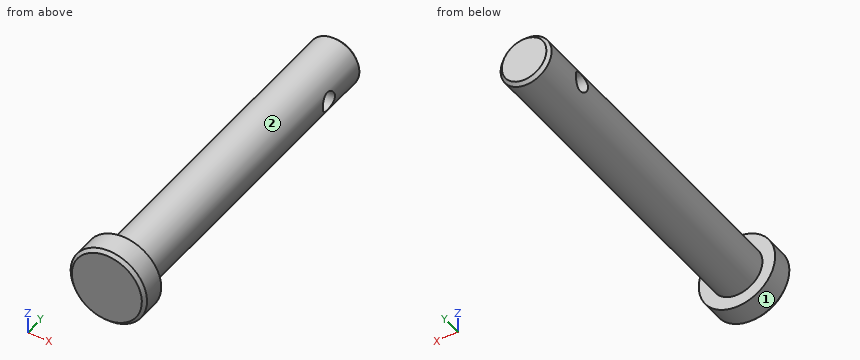
```python
from build123d import *

# Parameters (mm, degrees)
SKETCH1_R               = 12
BOSS_EXTRUDE1_DEPTH     = 8
CHAMFER1_SIZE           = 1
SKETCH2_R               = 8
BOSS_EXTRUDE2_DEPTH     = 105
CHAMFER2_SIZE           = 1
CUT_EXTRUDE1_DEPTH      = 115.267230648
CUT_EXTRUDE1_DEPTH_BACK = 115.267230648
SKETCH3_R               = 3


with BuildPart() as part:
    # Sketch1 → Boss-Extrude1 (new body)
    with BuildSketch(Plane(origin=(0, 0, 0), x_dir=(-1, 0, 0), z_dir=(0, 1, 0))):
        with Locations(Location((0, 0, 0), (0, 0, 90))):
            Circle(SKETCH1_R)
    extrude(amount=BOSS_EXTRUDE1_DEPTH)

    # Chamfer1
    chamfer1_edges = [part.edges().sort_by_distance(p)[0] for p in [
        (0, 0, -12),
    ]]
    chamfer(chamfer1_edges, length=CHAMFER1_SIZE)

    # Sketch2 → Boss-Extrude2 (add)
    with BuildSketch(Plane(origin=(0, 8, 0), x_dir=(-1, 0, 0), z_dir=(0, 1, 0))):
        with Locations(Location((0, 0, 0), (0, 0, 90))):
            Circle(SKETCH2_R)
    extrude(amount=BOSS_EXTRUDE2_DEPTH)

    # Chamfer2
    chamfer2_edges = [part.edges().sort_by_distance(p)[0] for p in [
        (0, 113, -8),
    ]]
    chamfer(chamfer2_edges, length=CHAMFER2_SIZE)

    # Sketch3 → Cut-Extrude1 (cut, two sides: drawn at the far end of the back side and taken through both)
    with BuildSketch(Plane.YZ.offset(-CUT_EXTRUDE1_DEPTH_BACK)):
        with Locations(Location((97, 0, 0), (0, 0, 270))):
            Circle(SKETCH3_R)
    extrude(amount=CUT_EXTRUDE1_DEPTH + CUT_EXTRUDE1_DEPTH_BACK, mode=Mode.SUBTRACT)


solid = part.part
```
Work out the finished part from the listing and answer in its coordinate system (mm). Face numbers are marked on the shaded views. A direction names the side the tool comes from. Give positions to 0.01 mm unless a question says otherwise; leave off trailing zeros. Loops run counter-clockwise (first coordinate to the right, second up) from the corner with the lowest first, then second, coordinate; pieces in that order, holes last. Notation, with made-up numbers: (7.25, 30) -> (16.25, 30) arc R31 cw to (16.25, 58) -> close; hole circle Ø3 at (-34, 42.25). An arc over 180 degrees is marked (long way). Use CSV: the item, a comma, the result in double quotes.
1. The part is cut by section C-C (y = 97). Write down the section's boundary in (x, z).
Found:
outline,"(-7.42, -3) arc R8 ccw to (7.42, -3) -> close; (-7.42, 3) -> (7.42, 3) arc R8 ccw to start"
2. Flat-ended cylindrical pins translate along their axes: pin 1 Ø1 at (y, z) = (93, 1) entering from -X; pin 2 Ø8 at (y, z) = (97, 0) entering from +X; pin 3 Ø4 at (x, y) = (5.5, 41) entering from -Z. Find the tip coordinate at first contact, or state that the pin passes through.
Found:
pin 1,"x = -7.98"
pin 2,"x = 8"
pin 3,"z = -7.19"
3. Straight lines are drawn through the part: line 1 (Y direction, x = -1, z = 0); line 2 (Y direction, x = -8, z = -7); line 3 (Y direction, x = 7.25, z = 2). For each, find the intervals that lie inside material, in ascending order.
Found:
line 1,"0 to 94, 100 to 113"
line 2,"0 to 8"
line 3,"0 to 94.76, 99.24 to 112.48"
4. A tool of negligible diameter and unlimited length cuts with its end or side. For the marked faces 1 and 2, from which of +Z, -Z, +X, -X, +Y, -Y can it reach the whole face along a straight path? Write none if from no direction.
Found:
face 1,"+Y, -Y"
face 2,"+Y"
5. The part is cut by section A-A (z = 0). Write down the section's boundary in (x, y).
Found:
outline,"(-12, 1) -> (-11, 0) -> (11, 0) -> (12, 1) -> (12, 8) -> (8, 8) -> (8, 94) -> (-8, 94) -> (-8, 8) -> (-12, 8) -> close; (-8, 100) -> (8, 100) -> (8, 112) -> (7, 113) -> (-7, 113) -> (-8, 112) -> close"
6. The part is cut by section B-B (x = 0). Write down the section's boundary in (y, z), then the cut area to 3 significant figures.
Found:
outline,"(0, -11) -> (1, -12) -> (8, -12) -> (8, -8) -> (112, -8) -> (113, -7) -> (113, 7) -> (112, 8) -> (8, 8) -> (8, 12) -> (1, 12) -> (0, 11) -> close; hole circle Ø6 at (97, 0)"
area,"1,840 mm^2"
